The drawing under review shows one solid part. Ordinate dimensions are in mm from its lowest x, y, z. A direction names the side the tool comes from. Coordinates: 2 decimals unless noted, no trailing zeros. Write each loop counter-clockwise with the first axis right and the second up, starting at its lowest first coordinate (ties: lowest second). Pieces come first, ordered by that corner, then holes.
Q1. Add section A-A, the plane x = 7. Give the boundary of the cut face in (y, z).
Q2. Add section D-D, the plane z = 1.5. Give the boundary of the cut face in (x, y).
Q3. The part is to be moulded in two halves that separate along X. For the marked faces 4, 5, 6 and 7, say which applies: +X half, -X half, draft (parallel to the pull), parting line (faces both ways), or undercut.
Q4. Add section B-B, the plane z = 7. Give the boundary of the cut face in (x, y).
Q5. Add section C-C, the plane y = 13.5. Give the boundary of the cut face in (x, z).
Q6. To check wall thickness, follow probe 1 along X at (y, z) = (1, 3.5); probe 2 along Z at (x, y) = (7, 14.55). State the ranges of each line that lie inside material, in increasing order.
Q7. Clearance check with flat-ended pins moving along their axes: pin 1 Ø8 at (x, z) = (3.5, 2) entering from +Y; pin 2 Ø4 at (x, y) = (11, 17.5) entering from +Z; pin 3 Ø0.5 at (y, z) = (14.5, 6.5) entering from -X; pin 4 Ø3 at (x, y) = (6, 17.5) entering from +Z. State where each tip first meets the part, or that it passes through.
Q8. Machinability: for the marked faces 1, 2 and 3, which of the approach directions +Z, -Z, +X, -X, +Y, -Y give a long, thin tool a straight path to every point of the face, cutting with its end or side? Answer none if there is none.
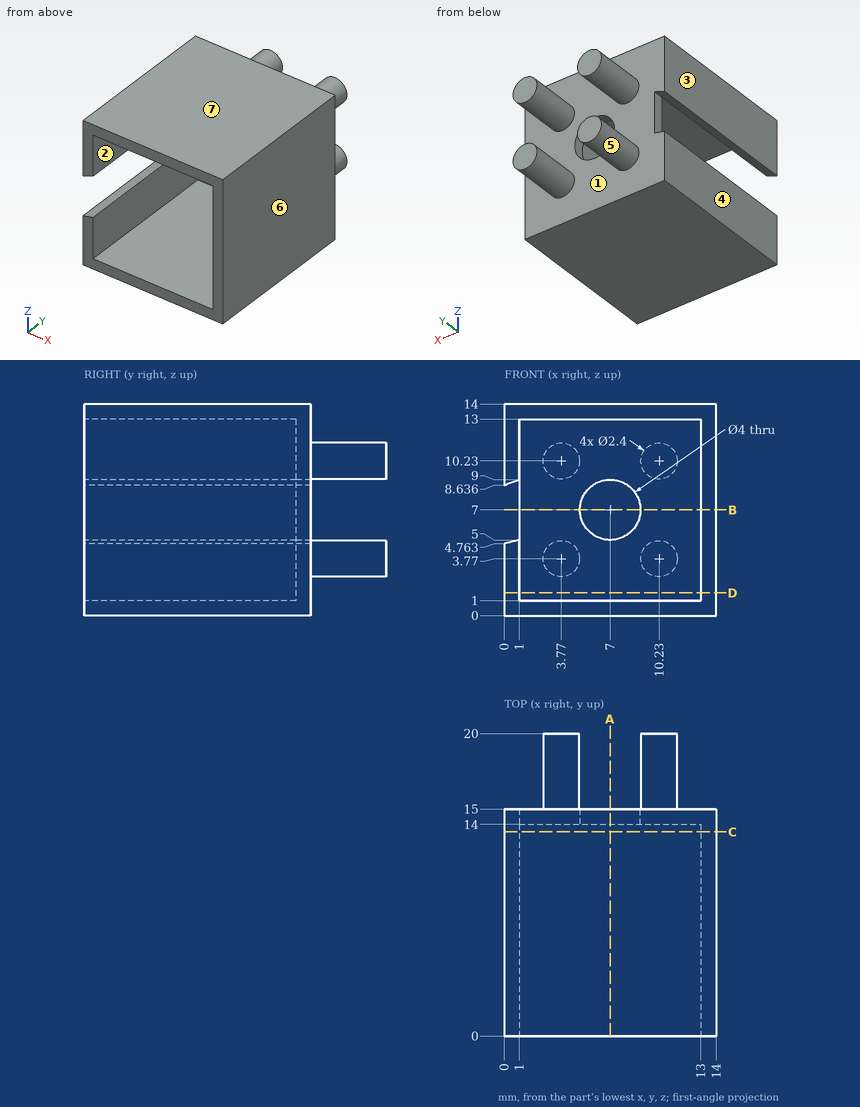
Here are the results:
1. outline: (0, 0) - (15, 0) - (15, 5) - (14, 5) - (14, 1) - (0, 1) - close; (0, 13) - (14, 13) - (14, 9) - (15, 9) - (15, 14) - (0, 14) - close
2. outline: (0, 0) - (1, 0) - (1, 14) - (13, 14) - (13, 0) - (14, 0) - (14, 15) - (0, 15) - close
3. face 4: -X half
3. face 5: undercut
3. face 6: +X half
3. face 7: draft
4. outline: (1, 14) - (5, 14) - (5, 15) - (1, 15) - close; (9, 14) - (13, 14) - (13, 0) - (14, 0) - (14, 15) - (9, 15) - close
5. outline: (0, 0) - (14, 0) - (14, 14) - (0, 14) - (0, 8.64) - (1, 9) - (1, 13) - (13, 13) - (13, 1) - (1, 1) - (1, 5) - (0, 4.76) - close
6. probe 1: x = 0 to 1, 13 to 14
6. probe 2: z = 0 to 5, 9 to 14
7. pin 1: stops at y = 20
7. pin 2: stops at z = 11.43
7. pin 3: stops at x = 1
7. pin 4: stops at z = 11.18
8. face 1: +Y
8. face 2: -Y
8. face 3: +Z, -Z, -X, +Y, -Y
